Part model, mm, in its own coordinate system. Face numbers are marked on the shaded views. Give positions to 0.01 mm unless a question says otherwise; leave off trailing zeros. Loops run counter-clockwise (first coordinate to the right, second up) from the corner with the lowest first, then second, coordinate; pieces in that order, holes last. Notation, with made-up numbers: (41.25, -6) -> (79.25, -6) arc R30 cw to (79.25, 21) -> close; hole circle Ø3 at (26.5, -20.75). An arc over 180 degrees is marked (long way). Write item = value, one per line.
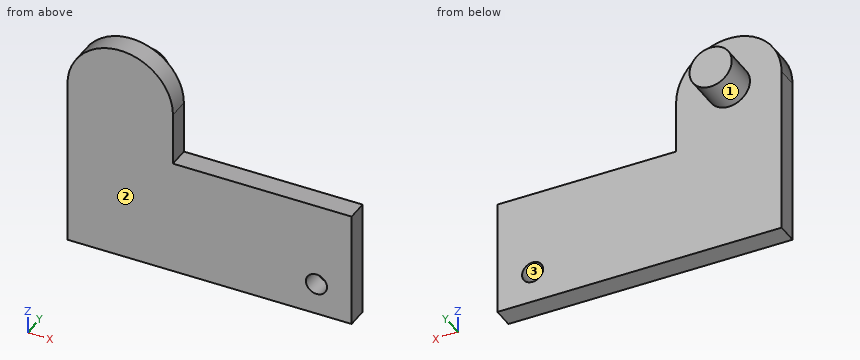
Autodesk Inventor part; units mm, degrees
ref_plane "YZ Plane" through (0, 0, 0) normal (1, 0, 0) x (0, 1, 0)
ref_plane "XZ Plane" through (0, 0, 0) normal (0, 1, 0) x (-1, 0, 0)
ref_plane "XY Plane" through (0, 0, 0) normal (0, 0, 1) x (1, 0, 0)
sketch "Sketch3" plane through (0, 0, 0) normal (0, 1, 0) x (-1, 0, 0)
  line L0 (0, 0) -> (0, -60)
  line L1 (0, 0) -> (60, 0) construction
  line L2 (0, -60) -> (12.519, -60)
  line L3 (0, 0) -> (25.4, 0)
  line L4 (25.4, 0) -> (25.4, 7.5)
  line L5 (25.4, 7.5) -> (40.4, 7.5)
  circle A0 centre (32.9, 7.5) radius 7.5
  circle A1 centre (32.9, 7.5) radius 3
  line L6 (40.4, 7.5) -> (40.4, -16.519)
  line L7 (40.4, -16.519) -> (12.519, -60)
  line L8 (0, -30) -> (5, -30)
  line L9 (5, -60) -> (5, -48)
  line L10 (5, 0) -> (5, -12)
  circle A2 centre (5, -12) radius 1.5
  circle A3 centre (5, -48) radius 1.5
  dimension "d6" = 60
  dimension "d7" = 90
  dimension "d8" = 12.519
  dimension "d9" = 25.4
  dimension "d10" = 7.5
  dimension "d11" = 15
  dimension "d12" = 6
  dimension "d13" = 24.019
  dimension "d18" = 5
  dimension "d19" = 12
  dimension "d20" = 12
  dimension "d21" = 3
  dimension "d22" = 3
extrude "Extrusion1" add sketch "Sketch3" along normal blind 3 contours L3 L4 A0 L6 L7 L2 L0 | A0 L5 A1 | L5 A1 A0 | L5 A1 picked at (33.8145, 6.796)
sketch "Sketch4" plane through (0, 0, 0) normal (0, -1, 0) x (1, 0, 0)
  line L0 (-35.9, 7.5) -> (-29.9, 7.5)
  line L1 (-29.9, 7.5) -> (-35.9, 7.5)
  circle A0 centre (-32.9, 7.5) radius 3
  point P0 (0, 0)
extrude "Extrusion2" add sketch "Sketch4" against normal blind 8
sketch "Sketch5" plane through (0, 3, 0) normal (0, 1, 0) x (1, 0, 0)
  line L0 (-40.4, 16.519) -> (-40.4, -7.5)
  line L1 (0, 60) -> (-12.519, 60)
  line L2 (-40.4, 60) -> (0, 60)
  line L3 (0, 60) -> (0, 16.519)
  line L4 (0, 16.519) -> (-40.4, 16.519)
  line L5 (-40.4, 16.519) -> (-40.4, 60)
  point P0 (0, 0)
extrude "Extrusion3" cut sketch "Sketch5" against normal blind 25.4
properties part number "exShortShaft"
1) Slice it at C-C, the plane y = 2.5. List the corners of the cut face in (x, z), and give its area (3 significant figures).
Resolved:
outline = (-40.4, -16.52) -> (0, -16.52) -> (0, 0) -> (-25.4, 0) -> (-25.4, 7.5) arc R7.5 ccw to (-40.4, 7.5) -> close; hole circle Ø3 at (-5, -12)
area = 861 mm²
2) Slice it at A-A, the plane z = -12. List the corners of the cut face in (x, y), and give its area (3 significant figures).
Resolved:
outline = (-40.4, 0) -> (-6.5, 0) -> (-6.5, 3) -> (-40.4, 3) -> close; (-3.5, 0) -> (0, 0) -> (0, 3) -> (-3.5, 3) -> close
area = 112 mm²
3) Pull direction Z, two halves, no side cores. Call the marked faces 1, 2 and 3: pulls with the +Z half, pulls with the -Z half, needs draft (parallel to the pull), parting line crosses it, or undercut.
Resolved:
face_1 = parting line crosses it
face_2 = needs draft
face_3 = undercut
4) Slice it at B-B, the plane x = -5. List the corners of the cut face in (y, z), and give its area (3 significant figures).
Resolved:
outline = (0, -16.52) -> (3, -16.52) -> (3, -13.5) -> (0, -13.5) -> close; (0, -10.5) -> (3, -10.5) -> (3, 0) -> (0, 0) -> close
area = 40.6 mm²
5) Drill centre lines: line 1 along X through (y, z) = (0.85, -12); line 2 along Z through (x, y) = (-5, 2); line 3 along Z through (x, y) = (-20, 0.75). Where is each one in solid material? Low to high. Write a range as [from, to].
Resolved:
line_1 = [-40.4, -6.5], [-3.5, 0]
line_2 = [-16.52, -13.5], [-10.5, 0]
line_3 = [-16.52, 0]
6) Slice it at D-D, the plane x = -32.9. List the corners of the cut face in (y, z), and give its area (3 significant figures).
Resolved:
outline = (0, -16.52) -> (3, -16.52) -> (3, 4.5) -> (8, 4.5) -> (8, 10.5) -> (3, 10.5) -> (3, 15) -> (0, 15) -> close
area = 125 mm²
7) Drop flat-ended pins along their axis: P1, Ø3.5, axis at x = -5, z = -12, coming from the +Y side; P2, Ø0.9, axis at y = 2, z = 4, coming from the +X side; P3, Ø2.5, axis at x = -18.5, y = 2, coming from the +Z side. Give the stop position or say it passes through.
Resolved:
P1 = 3
P2 = -25.4
P3 = 0
